from build123d import *

# Parameters (mm, degrees)
SPUR_START             = -34.432979129
SPUR_GEAR_AI_OUTLINE_R = 4.7625
SPUR_GEAR_AI_DEPTH     = 13.97
CUT_EXTRUDE1_DEPTH     = 34.814807958


# Read off the part's stored shape, not the designer's step: spur gear_ai
with BuildPart() as part:
    # spur gear_ai outline → spur gear_ai (new body)
    with BuildSketch(Plane.YZ.offset(SPUR_START)):
        with BuildLine():
            ThreePointArc((13.280785394, 8.759491053), (13.513878524, 9.095188342), (13.734821499, 9.439004105))
            ThreePointArc((13.734821499, 9.439004105), (12.859979854, 10.643431253), (11.610114863, 11.452028906))
            ThreePointArc((11.610114863, 11.452028906), (11.941871418, 12.159942302), (12.207854471, 12.895099975))
            ThreePointArc((12.207854471, 12.895099975), (13.663407365, 12.583076847), (15.133672429, 12.816128991))
            ThreePointArc((15.133672429, 12.816128991), (15.220556611, 13.215473725), (15.293108707, 13.617669288))
            ThreePointArc((15.293108707, 13.617669288), (14.023946102, 14.395627475), (12.559784493, 14.664371671))
            ThreePointArc((12.559784493, 14.664371671), (12.595380856, 15.445356105), (12.559784493, 16.22634054))
            ThreePointArc((12.559784493, 16.22634054), (14.023946102, 16.495084736), (15.293108707, 17.273042923))
            ThreePointArc((15.293108707, 17.273042923), (15.220556611, 17.675238486), (15.133672429, 18.07458322))
            ThreePointArc((15.133672429, 18.07458322), (13.663407365, 18.307635364), (12.207854471, 17.995612236))
            ThreePointArc((12.207854471, 17.995612236), (11.941871418, 18.730769909), (11.610114863, 19.438683305))
            ThreePointArc((11.610114863, 19.438683305), (12.859979854, 20.247280957), (13.734821499, 21.451708106))
            ThreePointArc((13.734821499, 21.451708106), (13.513878524, 21.795523869), (13.280785394, 22.131221158))
            ThreePointArc((13.280785394, 22.131221158), (11.8332524, 21.783887183), (10.607902954, 20.938599424))
            ThreePointArc((10.607902954, 20.938599424), (10.080833993, 21.516009243), (9.503424174, 22.043078204))
            ThreePointArc((9.503424174, 22.043078204), (10.348711933, 23.26842765), (10.696045908, 24.715960644))
            ThreePointArc((10.696045908, 24.715960644), (10.360348619, 24.949053774), (10.016532856, 25.169996749))
            ThreePointArc((10.016532856, 25.169996749), (8.812105708, 24.295155104), (8.003508055, 23.045290113))
            ThreePointArc((8.003508055, 23.045290113), (7.295594659, 23.377046668), (6.560436986, 23.643029721))
            ThreePointArc((6.560436986, 23.643029721), (6.872460114, 25.098582615), (6.63940797, 26.568847679))
            ThreePointArc((6.63940797, 26.568847679), (6.240063236, 26.65573186), (5.837867673, 26.728283957))
            ThreePointArc((5.837867673, 26.728283957), (5.059909486, 25.459121352), (4.79116529, 23.994959743))
            ThreePointArc((4.79116529, 23.994959743), (4.010180856, 24.030556105), (3.229196421, 23.994959743))
            ThreePointArc((3.229196421, 23.994959743), (2.960452225, 25.459121352), (2.182494038, 26.728283957))
            ThreePointArc((2.182494038, 26.728283957), (1.780298475, 26.65573186), (1.380953741, 26.568847679))
            ThreePointArc((1.380953741, 26.568847679), (1.147901597, 25.098582615), (1.459924725, 23.643029721))
            ThreePointArc((1.459924725, 23.643029721), (0.724767052, 23.377046668), (0.016853656, 23.045290113))
            ThreePointArc((0.016853656, 23.045290113), (-0.791743997, 24.295155104), (-1.996171145, 25.169996749))
            ThreePointArc((-1.996171145, 25.169996749), (-2.339986908, 24.949053774), (-2.675684197, 24.715960644))
            ThreePointArc((-2.675684197, 24.715960644), (-2.328350222, 23.26842765), (-1.483062463, 22.043078204))
            ThreePointArc((-1.483062463, 22.043078204), (-2.060472282, 21.516009243), (-2.587541243, 20.938599424))
            ThreePointArc((-2.587541243, 20.938599424), (-3.812890689, 21.783887183), (-5.260423683, 22.131221158))
            ThreePointArc((-5.260423683, 22.131221158), (-5.493516813, 21.795523869), (-5.714459788, 21.451708106))
            ThreePointArc((-5.714459788, 21.451708106), (-4.839618143, 20.247280957), (-3.589753152, 19.438683305))
            ThreePointArc((-3.589753152, 19.438683305), (-3.921509707, 18.730769909), (-4.18749276, 17.995612236))
            ThreePointArc((-4.18749276, 17.995612236), (-5.643045654, 18.307635364), (-7.113310718, 18.07458322))
            ThreePointArc((-7.113310718, 18.07458322), (-7.200194899, 17.675238486), (-7.272746996, 17.273042923))
            ThreePointArc((-7.272746996, 17.273042923), (-6.003584391, 16.495084736), (-4.539422782, 16.22634054))
            ThreePointArc((-4.539422782, 16.22634054), (-4.575019144, 15.445356106), (-4.539422782, 14.664371671))
            ThreePointArc((-4.539422782, 14.664371671), (-6.003584391, 14.395627475), (-7.272746996, 13.617669288))
            ThreePointArc((-7.272746996, 13.617669288), (-7.200194899, 13.215473725), (-7.113310718, 12.816128991))
            ThreePointArc((-7.113310718, 12.816128991), (-5.643045654, 12.583076847), (-4.18749276, 12.895099975))
            ThreePointArc((-4.18749276, 12.895099975), (-3.921509707, 12.159942302), (-3.589753152, 11.452028906))
            ThreePointArc((-3.589753152, 11.452028906), (-4.839618143, 10.643431253), (-5.714459788, 9.439004105))
            ThreePointArc((-5.714459788, 9.439004105), (-5.493516813, 9.095188342), (-5.260423683, 8.759491053))
            ThreePointArc((-5.260423683, 8.759491053), (-3.812890689, 9.106825028), (-2.587541243, 9.952112787))
            ThreePointArc((-2.587541243, 9.952112787), (-2.060472282, 9.374702968), (-1.483062463, 8.847634007))
            ThreePointArc((-1.483062463, 8.847634007), (-2.328350222, 7.622284561), (-2.675684197, 6.174751567))
            ThreePointArc((-2.675684197, 6.174751567), (-2.339986908, 5.941658437), (-1.996171145, 5.720715462))
            ThreePointArc((-1.996171145, 5.720715462), (-0.791743997, 6.595557107), (0.016853656, 7.845422098))
            ThreePointArc((0.016853656, 7.845422098), (0.724767052, 7.513665543), (1.459924725, 7.24768249))
            ThreePointArc((1.459924725, 7.24768249), (1.147901597, 5.792129596), (1.380953741, 4.321864532))
            ThreePointArc((1.380953741, 4.321864532), (1.780298475, 4.23498035), (2.182494038, 4.162428254))
            ThreePointArc((2.182494038, 4.162428254), (2.960452225, 5.431590859), (3.229196421, 6.895752468))
            ThreePointArc((3.229196421, 6.895752468), (4.010180855, 6.860156105), (4.79116529, 6.895752468))
            ThreePointArc((4.79116529, 6.895752468), (5.059909486, 5.431590859), (5.837867673, 4.162428254))
            ThreePointArc((5.837867673, 4.162428254), (6.240063236, 4.23498035), (6.63940797, 4.321864532))
            ThreePointArc((6.63940797, 4.321864532), (6.872460114, 5.792129596), (6.560436986, 7.24768249))
            ThreePointArc((6.560436986, 7.24768249), (7.295594659, 7.513665543), (8.003508055, 7.845422098))
            ThreePointArc((8.003508055, 7.845422098), (8.812105708, 6.595557107), (10.016532856, 5.720715462))
            ThreePointArc((10.016532856, 5.720715462), (10.360348619, 5.941658437), (10.696045908, 6.174751567))
            ThreePointArc((10.696045908, 6.174751567), (10.348711933, 7.622284561), (9.503424174, 8.847634007))
            ThreePointArc((9.503424174, 8.847634007), (10.080833993, 9.374702968), (10.607902954, 9.952112787))
            ThreePointArc((10.607902954, 9.952112787), (11.8332524, 9.106825028), (13.280785394, 8.759491053))
        make_face()
        with Locations((4.010180856, 15.445356105)):
            Circle(SPUR_GEAR_AI_OUTLINE_R, mode=Mode.SUBTRACT)
    extrude(amount=SPUR_GEAR_AI_DEPTH)

    # Sketch1 → Cut-Extrude1 (cut, through all)
    with BuildSketch(Plane(origin=(-20.462979129, 0, 0), x_dir=(0, 0, -1), z_dir=(1, 0, 0))):
        with BuildLine():
            Line((-13.445356105, 8.59275655), (-13.445356105, 11.010180856))
            Line((-13.445356105, 11.010180856), (-17.445356105, 11.010180856))
            Line((-17.445356105, 11.010180856), (-17.445356105, 8.59275655))
            ThreePointArc((-17.445356105, 8.59275655), (-15.445356105, 9.010180856), (-13.445356105, 8.59275655))
        make_face()
        with BuildLine():
            ThreePointArc((-10.445356105, 4.010180856), (-11.262055973, 6.748793643), (-13.445356105, 8.59275655))
            Line((-13.445356105, 8.59275655), (-13.445356105, 7.010180856))
            Line((-13.445356105, 7.010180856), (-17.445356105, 7.010180856))
            Line((-17.445356105, 7.010180856), (-17.445356105, 8.59275655))
            ThreePointArc((-17.445356105, 8.59275655), (-18.183968893, -0.173119277), (-10.445356105, 4.010180856))
        make_face()
        with BuildLine():
            Line((-13.445356105, 7.010180856), (-13.445356105, 8.59275655))
            ThreePointArc((-13.445356105, 8.59275655), (-15.445356105, 9.010180856), (-17.445356105, 8.59275655))
            Line((-17.445356105, 8.59275655), (-17.445356105, 7.010180856))
            Line((-17.445356105, 7.010180856), (-13.445356105, 7.010180856))
        make_face()
    extrude(amount=-CUT_EXTRUDE1_DEPTH, mode=Mode.SUBTRACT)


solid = part.part
Model file for the job. Use its own axes, mm. Coordinates: 2 decimals unless noted, no trailing zeros. Order: outer loops, then holes, each group sorted by start corner. A loop starts at its lowest first (then second) coordinate and runs counter-clockwise, first axis right, second up. Notation, with made-up numbers: M 11,-11.75 L 62,-11.75 A29 ccw 62,11.25 Z; hole C -20.5,37.25 d7. An arc over 180 degrees is marked long. Return JSON: item names as keys, results as strings.
1. Saw through at B-B (y = 0.5). Give the cut face in (x, z).
Ans:
{"outline": "M -34.43,7.61 L -20.46,7.61 L -20.46,11.88 L -34.43,11.88 Z; M -34.43,19.01 L -20.46,19.01 L -20.46,23.28 L -34.43,23.28 Z"}
2. Drill centre lines: probe 1 along Z at (x, y) = (-22.75, 13.5); probe 2 along Z at (x, y) = (-27.5, 11.75); probe 3 along Z at (x, y) = (-25.75, 4.75). Where is each one in solid material? Low to high.
Ans:
{"probe 1": "9.07 to 9.86, 12.59 to 14.56, 16.33 to 18.3, 21.03 to 21.82", "probe 2": "9.15 to 11.39, 11.73 to 19.16, 19.5 to 21.75", "probe 3": "6.89 to 10.5, 20.39 to 24"}
3. Saw through at C-C (z = 21.75). Give the cut face in (x, y).
Ans:
{"outline": "M -34.43,-5.52 L -20.46,-5.52 L -20.46,-3.74 L -34.43,-3.74 Z; M -34.43,-1.82 L -20.46,-1.82 L -20.46,9.84 L -34.43,9.84 Z; M -34.43,11.76 L -20.46,11.76 L -20.46,13.54 L -34.43,13.54 Z"}
4. Saw through at A-A (z = 15). Give the cut face in (x, y), and give its area (3 significant figures).
Ans:
{"outline": "M -34.43,-4.56 L -20.46,-4.56 L -20.46,-0.97 L -34.43,-0.97 Z; M -34.43,11.01 L -20.46,11.01 L -20.46,12.58 L -34.43,12.58 Z", "area": "72.2 mm^2"}
5. Flat gauge pins, fed straight in: pin 1 (2.5 mm diameter, centred on x = -27, y = 10, fed in from +Z); pin 2 (5 mm diameter, centred on x = -29.5, z = 11, fed in from +Y); pin 3 (1.5 mm diameter, centred on x = -27, y = 8.5, fed in from +Z). Where does each tip first touch, or does it go through?
Ans:
{"pin 1": "z = 25.17", "pin 2": "y = 15.27", "pin 3": "z = 24.69"}
6. Pull direction Z, two halves, no side cores. Call faces 1 (the face through (-27.546, -2.068, 9.382)), 2 (the face through (-27.546, 6.234, 4.234)), 3 (the face through (-27.55, -2.34, 23.29)): +Z half, -Z half, draft (parallel to the pull), parting line (faces both ways), or undercut.
Ans:
{"face 1": "undercut", "face 2": "-Z half", "face 3": "undercut"}
